The figure shows three views and two pictorial views of one solid part (mm, origin at its lowest corner). Answer the questions. A direction names the side the tool comes from. Give positions to 0.01 mm unless a question says otherwise; leave off trailing zeros. Order: outer loops, then holes, each group sorted by start corner. A loop starts at its lowest first (then second) coordinate and runs counter-clockwise, first axis right, second up. Notation, with made-up numbers: (47.25, 39.25) - (95.25, 39.25) arc R18 cw to (95.25, 47.25) - close; hole circle Ø7 at (-10, 13). An arc over 180 degrees is marked (long way). Answer as CSV lines item,"result". Start each with the question number.
1. Which of the six approach directions +Z, -Z, +X, -X, +Y, -Y give full straight-line access (tool end or side, diameter ignored) to the marked faces 1, 2 and 3?
2. Consider line 1 along Y through (x, z) = (44.5, 6.5); line 2 along X through (y, z) = (2.5, 17); line 3 along X through (y, z) = (3, 15). Determine where each line is inside the solid, lowest interval first. Write a range as [from, to].
3. Flat-ended cylindrical pins translate along their axes: pin 1 (1.5 mm diameter, centred on y = 11.5, z = 13.5, fed in from +X); pin 2 (4 mm diameter, centred on x = 21.5, y = 8, fed in from +Z); pin 3 (6.5 mm diameter, centred on x = 42, y = 19, fed in from +Z). Find the tip coordinate at first contact, or state that the pin passes through.
4. Section A-A on x = 38.5 is taken. Give the vertices of the cut face in (y, z).
5. Section D-D on x = 26.5 is taken. Give the vertices of the cut face in (y, z), and give its area (3 significant figures).
6. Section C-C on y = 8.25 is taken. Give the vertices of the cut face in (x, z), and give its area (3 significant figures).
7. Section B-B on z = 12 is taken. Give the vertices of the cut face in (x, y).
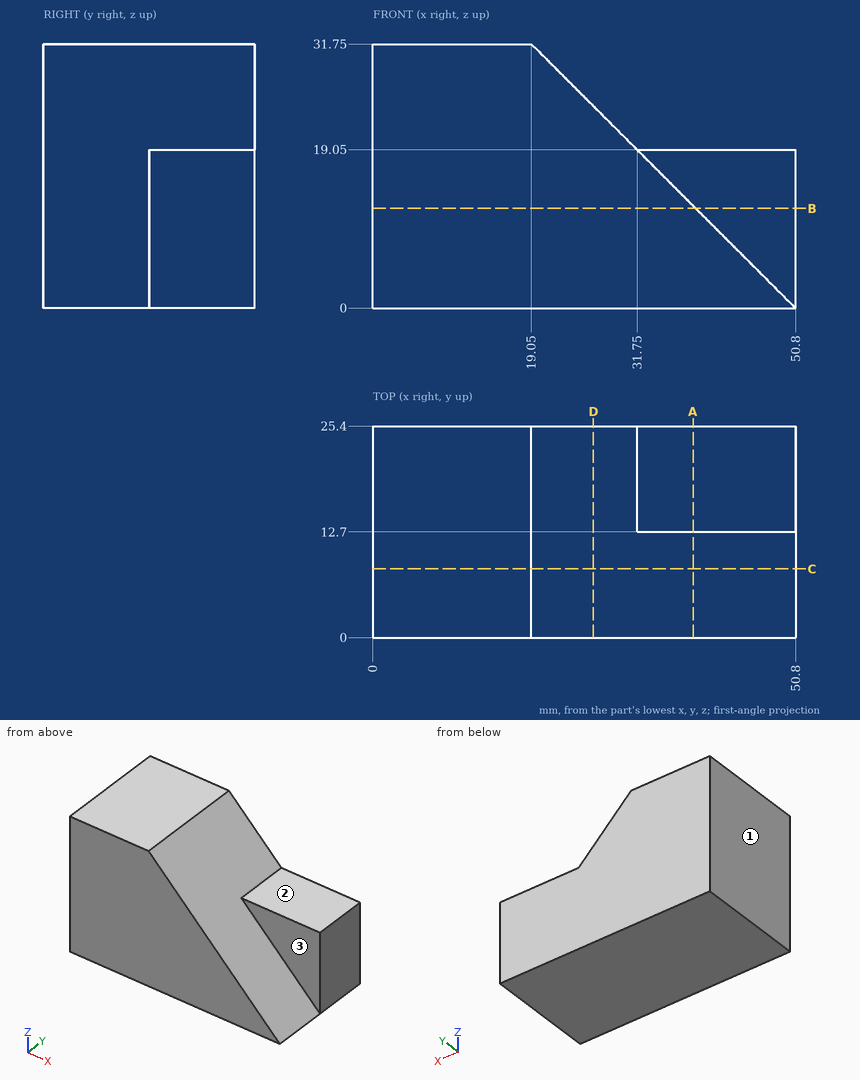
Checks:
1,face 1,"+Z, -Z, -X, +Y, -Y"
1,face 2,"+Z, +X, +Y, -Y"
1,face 3,"+Z, +X, -Y"
2,line 1,"y = [12.7, 25.4]"
2,line 2,"x = [0, 33.8]"
2,line 3,"x = [0, 35.8]"
3,pin 1,"stops at x = 38.05"
3,pin 2,"stops at z = 31.3"
3,pin 3,"stops at z = 19.05"
4,outline,"(0, 0) - (25.4, 0) - (25.4, 19.05) - (12.7, 19.05) - (12.7, 12.3) - (0, 12.3) - close"
5,outline,"(0, 0) - (25.4, 0) - (25.4, 24.3) - (0, 24.3) - close"
5,area,"617 mm²"
6,outline,"(0, 0) - (50.8, 0) - (19.05, 31.75) - (0, 31.75) - close"
6,area,"1,110 mm²"
7,outline,"(0, 0) - (38.8, 0) - (38.8, 12.7) - (50.8, 12.7) - (50.8, 25.4) - (0, 25.4) - close"
